from build123d import *

# Parameters (mm, degrees)
SKETCH1_W           = 122
SKETCH1_H           = 44
BOSS_EXTRUDE1_DEPTH = 1.6
SKETCH2_W           = 105.6
SKETCH2_H           = 34.2
BOSS_EXTRUDE2_DEPTH = 4.9
SKETCH3_R           = 1.75
CUT_EXTRUDE1_DEPTH  = 66.030838838
SKETCH5_W           = 99
SKETCH5_H           = 24
CUT_EXTRUDE2_DEPTH  = 1
SKETCH4_R           = 0.5
CUT_EXTRUDE3_DEPTH  = 66.030838838
LPATTERN1_COUNT     = 15
LPATTERN1_PITCH     = 2.54


with BuildPart() as part:
    # Sketch1 → Boss-Extrude1 (new body)
    with BuildSketch(Plane(origin=(0, 0, 0), x_dir=(1, 0, 0), z_dir=(0, 1, 0))):
        Rectangle(SKETCH1_W, SKETCH1_H)
    extrude(amount=BOSS_EXTRUDE1_DEPTH)

    # Sketch2 → Boss-Extrude2 (add)
    with BuildSketch(Plane(origin=(0, 1.6, 0), x_dir=(1, 0, 0), z_dir=(0, 1, 0))):
        with Locations((0, 1.3)):
            Rectangle(SKETCH2_W, SKETCH2_H)
    extrude(amount=BOSS_EXTRUDE2_DEPTH)

    # Sketch3 → Cut-Extrude1 (cut, through all)
    with BuildSketch(Plane(origin=(0, 1.6, 0), x_dir=(1, 0, 0), z_dir=(0, 1, 0))):
        with Locations(Location((-57.5, 18.5, 0), (0, 0, 270))):
            Circle(SKETCH3_R)
        with Locations(Location((-57.5, -18.5, 0), (0, 0, 270))):
            Circle(SKETCH3_R)
        with Locations(Location((57.5, 18.5, 0), (0, 0, 270))):
            Circle(SKETCH3_R)
        with Locations(Location((57.5, -18.5, 0), (0, 0, 270))):
            Circle(SKETCH3_R)
    extrude(amount=-CUT_EXTRUDE1_DEPTH, mode=Mode.SUBTRACT)

    # Sketch5 → Cut-Extrude2 (cut)
    with BuildSketch(Plane(origin=(0, 6.5, 0), x_dir=(1, 0, 0), z_dir=(0, 1, 0))):
        with Locations((0, 1.3)):
            Rectangle(SKETCH5_W, SKETCH5_H)
    extrude(amount=-CUT_EXTRUDE2_DEPTH, mode=Mode.SUBTRACT)

    # Sketch4 → Cut-Extrude3 (cut, through all)
    with BuildSketch(Plane(origin=(0, 1.6, 0), x_dir=(1, 0, 0), z_dir=(0, 1, 0))):
        with Locations(Location((-50.02, -19.5, 0), (0, 0, 270))):
            Circle(SKETCH4_R)
    cut_extrude3 = extrude(amount=-CUT_EXTRUDE3_DEPTH, mode=Mode.SUBTRACT)

    # LPattern1: Cut-Extrude3 ×15
    with Locations(*[(i * LPATTERN1_PITCH, 0, 0) for i in range(1, LPATTERN1_COUNT)]):
        add(cut_extrude3, mode=Mode.SUBTRACT)


solid = part.part
CAD build for the part. Positions are in the model's coordinates, mm. A direction names the side the tool comes from. Round coordinates to 2 decimals unless told otherwise and drop trailing zeros. Order: outer loops, then holes, each group sorted by start corner. A loop starts at its lowest first (then second) coordinate and runs counter-clockwise, first axis right, second up. Notation, with made-up numbers: (-19.5, -13.5) -> (-15.5, -13.5) arc R27 ccw to (-15.5, 7.5) -> close; hole circle Ø2 at (5, 59). An arc over 180 degrees is marked (long way). Write each question's results on one line, items separated by ' | '.
1. Cut at B-B (z = 7). Give the cut face in (x, y).
Findings below:
outline: (-61, 0) -> (61, 0) -> (61, 1.6) -> (52.8, 1.6) -> (52.8, 6.5) -> (49.5, 6.5) -> (49.5, 5.5) -> (-49.5, 5.5) -> (-49.5, 6.5) -> (-52.8, 6.5) -> (-52.8, 1.6) -> (-61, 1.6) -> close
2. Cut at A-A (x = 57.5). Give the cut face in (y, z), plus the area to 3 significant figures.
Findings below:
outline: (0, -22) -> (1.6, -22) -> (1.6, -20.25) -> (0, -20.25) -> close; (0, -16.75) -> (1.6, -16.75) -> (1.6, 16.75) -> (0, 16.75) -> close; (0, 20.25) -> (1.6, 20.25) -> (1.6, 22) -> (0, 22) -> close | area: 59.2 mm²
3. 3-axis set-ups, long thin cutter, end or side, ignore diameter. For faces 1 (the face through (-1, 4, 15.8)), 2 (the face through (-59.21, 0.81, -18.88)), 3 (the face through (52.8, 4, -1)): which of +Z, -Z, +X, -X, +Y, -Y reach the whole face in a straight line?
Findings below:
face 1: +Z, +X, -X, +Y | face 2: +Y, -Y | face 3: +Z, -Z, +X, +Y
4. Wall check: line 1 along Z through (x, y) = (-34.78, 0.65); line 2 along Z through (x, y) = (-1.5, 2); line 3 along X through (y, z) = (4, 7.5). Give the ranges that are in metal, low to high. Write a range as [from, to].
Findings below:
line 1: z = [-22, 19], [20, 22] | line 2: z = [-18.4, 15.8] | line 3: x = [-52.8, 52.8]
5. Cut at C-C (x = 8). Give the cut face in (y, z).
Findings below:
outline: (0, -22) -> (1.6, -22) -> (1.6, -18.4) -> (6.5, -18.4) -> (6.5, -13.3) -> (5.5, -13.3) -> (5.5, 10.7) -> (6.5, 10.7) -> (6.5, 15.8) -> (1.6, 15.8) -> (1.6, 22) -> (0, 22) -> close
6. Cut at D-D (y = 4.5). Give the cut face in (x, z).
Findings below:
outline: (-52.8, -18.4) -> (52.8, -18.4) -> (52.8, 15.8) -> (-52.8, 15.8) -> close
7. Pull direction Z, two halves, no side cores. Call faces 4 (the face through (-1, 4, -18.4)), 5 (the face through (-1, 5.5, -1)), 6 (the face through (-52.8, 4, -1)): pulls with the +Z half, pulls with the -Z half, needs draft (parallel to the pull), parting line crosses it, or undercut.
Findings below:
face 4: pulls with the -Z half | face 5: undercut | face 6: needs draft
8. Flat gauge pins, fed straight in: P1, Ø1.1, axis at x = -14.5, y = 6, coming from the -Z side; P2, Ø0.8, axis at y = 6, z = 3, coming from the -X side; P3, Ø1.5, axis at x = -38, z = -11.5, coming from the -Y side; P4, Ø1.1, axis at y = 6, z = 2, coming from the +X side. Where does each tip first touch, or does it go through?
Findings below:
P1: stops at z = -18.4 | P2: stops at x = -52.8 | P3: stops at y = 0 | P4: stops at x = 52.8
